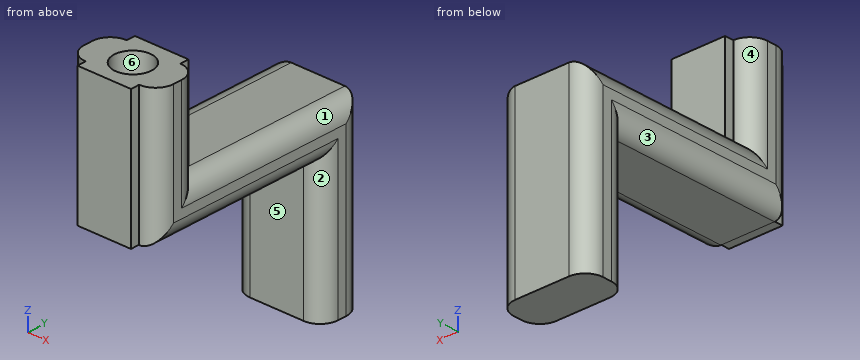
Autodesk Inventor part; units mm, degrees
ref_plane "YZ Plane" through (0, 0, 0) normal (1, 0, 0) x (0, 1, 0)
ref_plane "XZ Plane" through (0, 0, 0) normal (0, 1, 0) x (-1, 0, 0)
ref_plane "XY Plane" through (0, 0, 0) normal (0, 0, 1) x (1, 0, 0)
sketch "Sketch1" plane through (0, 0, 0) normal (1, 0, 0) x (0, 1, 0)
  line L0 (0, 0) -> (0, -10)
  line L1 (0, -10) -> (20, -10)
  line L2 (20, -10) -> (20, -30)
  line L3 (20, -30) -> (15, -30)
  line L4 (15, -30) -> (15, -15)
  line L5 (15, -15) -> (-5, -15)
  line L6 (-5, -15) -> (-5, 0)
  line L7 (-5, 0) -> (0, 0)
  dimension "d0" = 10
  dimension "d1" = 20
  dimension "d2" = 20
  dimension "d3" = 5
  dimension "d4" = 15
  dimension "d5" = 20
  dimension "d6" = 15
extrude "Extrusion1" add sketch "Sketch1" along normal blind 10
sketch "Sketch2" plane through (0, -5, 0) normal (0, 0, 1) x (1, 0, 0)
  line L0 (0, 0) -> (0, 5)
  line L1 (0, 5) -> (10, 5)
  point P0 (5, 2.5)
  dimension "d9" = 5
  dimension "d10" = 2.5
sketch "Sketch3" plane through (0, -5, 0) normal (0, 0, 1) x (1, 0, 0)
  circle A0 centre (5, 2.5) radius 2.0828
  line L0 (10, 5) -> (10, 0)
  line L1 (0, 5) -> (10, 5)
  dimension "d11" = 4.1656
  dimension "d12" = 5
  dimension "d13" = 2.5
extrude "Extrusion2" cut sketch "Sketch3" against normal blind 10
thread "Thread1"
fillet "Fillet1" radius 2 12 edges at (10, 20, -20) (0, 20, -20) (10, 0, -5) (0, 0, -5) (10, 15, -22.5) (10, -5, -7.5) (0, -5, -7.5) (0, 10, -10) (0, 5, -15) (10, 10, -10) (0, 15, -22.5) (10, 5, -15)
sketch "Sketch4" plane through (2, -5, -15) normal (0, -1, 0) x (1, 0, 0)
  line L0 (0, 15) -> (0, 5)
  line L1 (6, -15) -> (6, 5)
  line L2 (0, 15) -> (6, 15)
  line L3 (6, 15) -> (6, 0.0408)
  line L4 (6, 0.0408) -> (0, 0.0408)
  line L5 (0, 0.0408) -> (0, 15)
  point P0 (-2, 15)
extrude "Extrusion3" add sketch "Sketch4" along normal blind 1
sketch "Sketch5" plane through (2, 0, 0) normal (0, 1, 0) x (1, 0, 0)
  line L0 (6, 10) -> (6, 0)
  line L1 (0, 10) -> (6, 10)
  line L2 (6, 0) -> (0, 0)
  line L3 (0, 0) -> (0, 10)
  line L4 (0, 10) -> (6, 10)
  line L5 (6, 10) -> (6, 0)
  point P0 (-2, 0)
extrude "Extrusion4" add sketch "Sketch5" along normal blind 1
properties part number "Lever"
CAD build for the part. Positions are in the model's coordinates, mm. Face numbers are marked on the shaded views. A direction names the side the tool comes from. Coordinates: 2 decimals unless noted, no trailing zeros. Write each loop counter-clockwise with the first axis right and the second up, starting at its lowest first coordinate (ties: lowest second). Pieces come first, ordered by that corner, then holes. Notation, with made-up numbers: (58.25, 66.5) -> (98.25, 66.5) arc R17 ccw to (98.25, 87.5) -> close; hole circle Ø4 at (86.25, 61.5). An arc over 180 degrees is marked (long way). Use CSV: the item, a comma, the result in double quotes. Start each with the question number.
Item 1: Tool access for the marked faces 1, 2 and 3: list every direction of +Z, -Z, +X, -X, +Y, -Y with a clear straight run to the whole face (end or side of a thin tool).
Item 2: Band-saw the part on A-A, the plane z = -8.75. Write the cut outline in (x, y).
Item 3: Band-saw the part on D-D, the plane x = 5. Write the cut outline in (y, z).
Item 4: Band-saw the part on C-C, the plane z = -17.75. Write the cut outline in (x, y), plus the area to 3 significant figures.
Item 5: Two-plate mould, pull along Y, no slides. Class the marked faces 4, 5 and 6: +Y half, -Y half, draft (parallel to the pull), parting line (faces both ways), or undercut.
Item 6: Wall check: probe 1 along Y at (x, z) = (5, -3); probe 2 along Z at (x, y) = (2.75, -2.75); probe 3 along Y at (x, z) = (4, -19.5). Give the ranges that are in metal, low to high.
Item 7: Band-saw the part on B-B, the plane y = -2.5. Write the cut outline in (x, z).
Item 8: Drop flat-ended pins along their axis: P1, Ø1.1, axis at x = 4, y = -5.5, coming from the -Z side; P2, Ø3, axis at x = 3, y = 14, coming from the +Z side; P3, Ø5, axis at x = 4.5, z = -19.5, coming from the -Y side. Give the stop position or say it passes through.
Response values:
1,face 1,"+Z, +X, +Y"
1,face 2,"-Z, +X, -Y"
1,face 3,"-Z, -X, -Y"
2,outline,"(0, -3) arc R2 ccw to (2, -5) -> (2, -6) -> (8, -6) -> (8, -5) arc R2 ccw to (10, -3) -> (10, -2) arc R2 ccw to (8, 0) -> (8, 1) -> (2, 1) -> (2, 0) arc R2 ccw to (0, -2) -> close; hole circle Ø4.17 at (5, -2.5)"
3,outline,"(-6, -14.96) -> (-5, -14.96) -> (-5, -15) -> (15, -15) -> (15, -30) -> (20, -30) -> (20, -10) -> (1, -10) -> (1, 0) -> (-0.42, 0) -> (-0.42, -10) -> (-4.58, -10) -> (-4.58, 0) -> (-6, 0) -> close"
4,outline,"(0, 17) arc R2 ccw to (2, 15) -> (8, 15) arc R2 ccw to (10, 17) -> (10, 18) arc R2 ccw to (8, 20) -> (2, 20) arc R2 ccw to (0, 18) -> close"
4,area,"46.6 mm2"
5,face 4,"+Y half"
5,face 5,"-Y half"
5,face 6,"undercut"
6,probe 1,"y = -6 to -4.58, -0.42 to 1"
6,probe 2,"z = -15 to 0"
6,probe 3,"y = 15 to 20"
7,outline,"(0, -13) arc R2 ccw to (2, -15) -> (8, -15) arc R2 ccw to (10, -13) -> (10, 0) -> (7.08, 0) -> (7.08, -10) -> (2.92, -10) -> (2.92, 0) -> (0, 0) -> close"
8,P1,"stops at z = -15"
8,P2,"stops at z = -10"
8,P3,"stops at y = 15"
